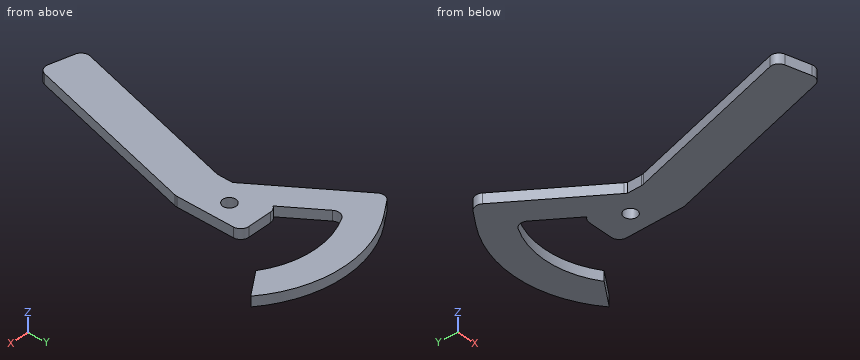
from build123d import *

# Parameters (mm, degrees)
MODEL_R             = 3.25
MODEL_R_2           = 2.075
BOSS_EXTRUDE1_DEPTH = 5


with BuildPart() as part:
    # Model → Boss-Extrude1 (new body)
    with BuildSketch(Plane.XY):
        with BuildLine():
            Line((299.530455157, 221.325483104), (287.530455157, 221.325483104))
            ThreePointArc((287.530455157, 221.325483104), (284.702028033, 220.153910229), (283.530455157, 217.325483104))
            Line((283.530455157, 217.325483104), (283.530455157, 191.852093095))
            ThreePointArc((283.530455157, 191.852093095), (283.496234603, 191.329988326), (283.394158462, 190.816816914))
            Line((283.394158462, 190.816816914), (261.272017278, 108.255862044))
            ThreePointArc((261.272017278, 108.255862044), (261.671618968, 105.220585863), (264.100444403, 103.356882558))
            Line((264.100444403, 103.356882558), (275.691554319, 100.251054017))
            ThreePointArc((275.691554319, 100.251054017), (278.726830499, 100.650655707), (280.590533804, 103.079481141))
            Line((280.590533804, 103.079481141), (303.394158462, 188.183766963))
            ThreePointArc((303.394158462, 188.183766963), (303.496234603, 188.696938374), (303.530455157, 189.219043143))
            Line((303.530455157, 189.219043143), (303.530455157, 217.325483104))
            ThreePointArc((303.530455157, 217.325483104), (302.358882282, 220.153910229), (299.530455157, 221.325483104))
        make_face()
        with Locations((293.530455157, 206.325483104)):
            Circle(MODEL_R, mode=Mode.SUBTRACT)
        with Locations((293.530455157, 214.325483104)):
            Circle(MODEL_R_2, mode=Mode.SUBTRACT)
        with Locations((293.530455157, 198.325483104)):
            Circle(MODEL_R_2, mode=Mode.SUBTRACT)
        with BuildLine():
            ThreePointArc((330.635106632, 250.251498618), (296.090916254, 263.768446459), (260.481102457, 253.378541305))
            Line((260.481102457, 253.378541305), (253.558218086, 248.516012577))
            ThreePointArc((253.558218086, 248.516012577), (251.917062939, 245.931599145), (252.584047269, 242.943670949))
            Line((252.584047269, 242.943670949), (282.759543213, 199.982183026))
            Line((282.759543213, 199.982183026), (283.508108229, 198.855371857))
            Line((283.508108229, 198.855371857), (283.530455157, 198.825483104))
            Line((283.530455157, 198.825483104), (283.530455157, 217.325483104))
            ThreePointArc((283.530455157, 217.325483104), (283.70765552, 218.5028543), (284.223556624, 219.575910195))
            Line((284.223556624, 219.575910195), (271.521515193, 237.660073602))
            ThreePointArc((271.521515193, 237.660073602), (270.895698021, 240.852034508), (272.848206871, 243.453566893))
            ThreePointArc((272.848206871, 243.453566893), (295.63531403, 248.773328387), (317.784347872, 241.225321044))
            Line((317.784347872, 241.225321044), (330.635106632, 250.251498618))
        make_face()
        with Locations((293.530455157, 198.325483104)):
            Circle(MODEL_R_2)
        with Locations((293.530455157, 214.325483104)):
            Circle(MODEL_R_2)
    extrude(amount=BOSS_EXTRUDE1_DEPTH)


solid = part.part
Part model, mm, in its own coordinate system. Give positions to 0.01 mm unless a question says otherwise; leave off trailing zeros. Order: outer loops, then holes, each group sorted by start corner. A loop starts at its lowest first (then second) coordinate and runs counter-clockwise, first axis right, second up. Notation, with made-up numbers: (-13, -19.75) - (1, -19.75) arc R17 ccw to (1, 5.25) - close; hole circle Ø4 at (-17, -9.5). An arc over 180 degrees is marked (long way). Use a Markdown table: item, result.
1) Probe L1, parallel to X at y = 220.5, z = 1.4; L2, parallel to X at y = 208, z = 2.75; L3, parallel to X at y = 120, z = 0.35. List the from-to ranges inside material, lowest first. Write a range as from..to.
Checked values:
| item | result |
|---|---|
| L1 | 268.35..283.57, 285.1..301.96 |
| L2 | 277.13..290.75, 296.32..303.53 |
| L3 | 264.42..285.12 |
2) Saw through at D-D on y = 122.5. List the corners of the cut face in (x, z), plus the area to 3 significant figures.
Checked values:
| item | result |
|---|---|
| outline | (265.09, 0) - (285.79, 0) - (285.79, 5) - (265.09, 5) - close |
| area | 104 mm² |
3) Flat gauge pins, fed straight in: P1, Ø2, axis at y = 126, z = 1, coming from the +X side; P2, Ø1, axis at x = 276, y = 226.5, coming from the -Z side; P3, Ø2.5, axis at y = 195, z = 1.5, coming from the -X side; P4, Ø4, axis at x = 293.53, y = 206.33, coming from the -Z side. Where does each tip first touch, or does it go through?
Checked values:
| item | result |
|---|---|
| P1 | x = 287 |
| P2 | z = 0 |
| P3 | x = 283.53 |
| P4 | through |
4) Saw through at C-C on x = 311. List the corners of the cut face in (y, z).
Checked values:
| item | result |
|---|---|
| outline | (245.07, 0) - (261.11, 0) - (261.11, 5) - (245.07, 5) - close |
5) Saw through at A-A on x = 292.5. List the corners of the cut face in (y, z), plus the area to 3 significant figures.
Checked values:
| item | result |
|---|---|
| outline | (147.53, 0) - (203.24, 0) - (203.24, 5) - (147.53, 5) - close; (209.41, 0) - (221.33, 0) - (221.33, 5) - (209.41, 5) - close; (248.81, 0) - (263.82, 0) - (263.82, 5) - (248.81, 5) - close |
| area | 413 mm² |
